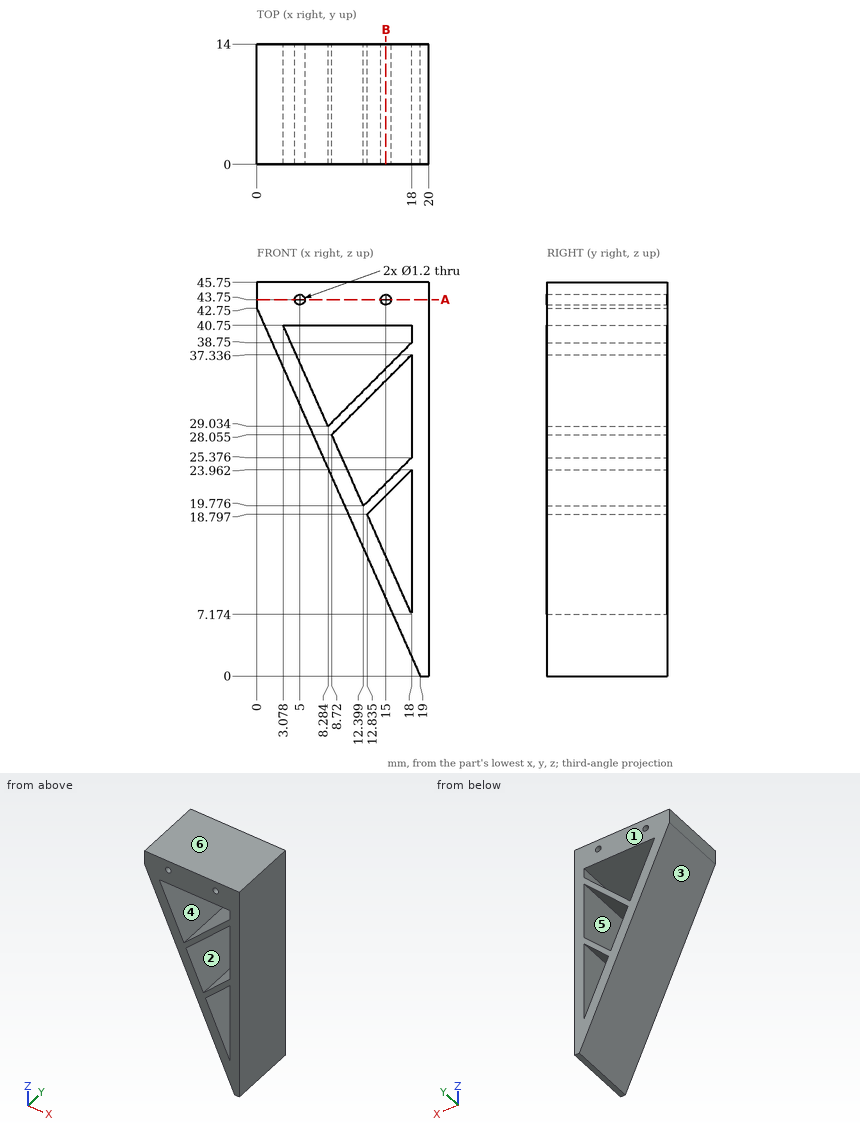
Could you check a few things on this drawing? It's one solid part, dimensions in mm from its lowest x, y, z. A direction names the side the tool comes from. Coordinates: 2 decimals unless noted, no trailing zeros. Order: outer loops, then holes, each group sorted by start corner. A loop starts at its lowest first (then second) coordinate and runs counter-clockwise, first axis right, second up. Notation, with made-up numbers: (-37.5, -7.5) - (-9.5, -7.5) arc R18 ccw to (-9.5, 9.5) - close; hole circle Ø6 at (-20.75, 37). An arc over 180 degrees is marked (long way). One line per question, with ' | ' between items. Start each with the question number.
1. I'm going to push flat-ended pins straight in: pin 1 Ø1.9 at (x, z) = (15, 43.75) entering from +Y; pin 2 Ø2 at (x, z) = (9, 19) entering from -Y; pin 3 Ø0.6 at (y, z) = (9.5, 39.5) entering from -X; pin 4 Ø6 at (y, z) = (9, 33) entering from -X. Where does each tip first touch, or does it pass through?
2. If we section it at B-B (x = 15): Give the number of separate pieces and of enclosed holes in the cut face, and give its area (3 significant figures).
3. Which directions (+Z, -Z, +X, -X, +Y, -Y) give clear straight access to the entire face, cutting with the end or side of a thin tool? Please do the marked faces 1 and 2.
4. If we section it at A-A (z = 43.75): Write out the boundary of the cut face in (x, y).
5. Please list where these lines run through material, in increasing order: line 1 along X through (y, z) = (10.5, 43.75); line 2 along X through (y, z) = (1, 21) (1 decimal); line 3 along X through (y, z) = (2.25, 18.5) (1 decimal). Write a range as [from, to].
6. If we mould it in two halves opening along X, with no side actions, what happens to the marked faces 3, 4, 5 and 6? For each: released by +X, released by -X, zero draft, split by the parting line, or undercut.
Model answer:
1) pin 1: stops at y = 14 | pin 2: passes through | pin 3: stops at x = 1.31 | pin 4: stops at x = 3
2) separate pieces: 5 | enclosed holes: 0 | area: 162 mm²
3) face 1: +Z, -Z, +X, -X, +Y | face 2: +Y, -Y
4) outline: (0, 0) - (4.4, 0) - (4.4, 14) - (0, 14) - close; (5.6, 0) - (14.4, 0) - (14.4, 14) - (5.6, 14) - close; (15.6, 0) - (20, 0) - (20, 14) - (15.6, 14) - close
5) line 1: x = [0, 4.4], [5.6, 14.4], [15.6, 20] | line 2: x = [9.7, 11.9], [13.6, 15], [18, 20] | line 3: x = [10.8, 13], [18, 20]
6) face 3: released by -X | face 4: undercut | face 5: undercut | face 6: zero draft
